Can you work these out from the model? Positions are in its coordinate system, mm. Face numbers are marked on the shaded views. Give positions to 0.01 mm unless a question says otherwise; leave off trailing zeros. Write each loop counter-clockwise with the first axis right and the second up, starting at its lowest first coordinate (ties: lowest second). Pieces come first, ordered by that corner, then holes.
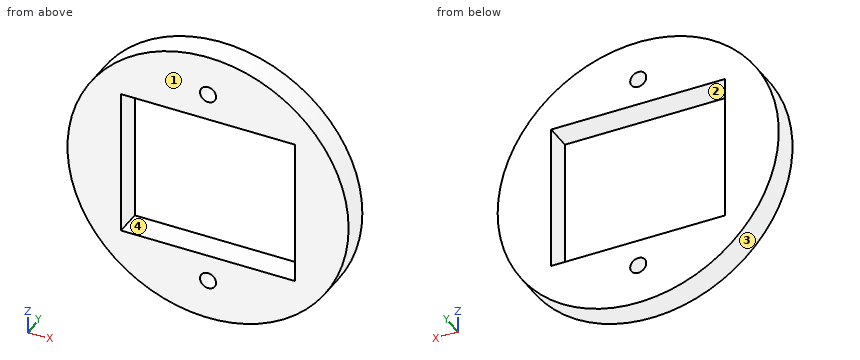
```python
from build123d import *

# Parameters (mm, degrees)
SKETCH1_R           = 26.67
SKETCH1_R_2         = 1.524
BOSS_EXTRUDE2_DEPTH = 5.08
SKETCH4_W           = 33.02
SKETCH4_H           = 27.94
CUT_EXTRUDE1_DEPTH  = 6.08


with BuildPart() as part:
    # Sketch1 → Boss-Extrude2 (new body)
    with BuildSketch(Plane(origin=(0, 0, 0), x_dir=(1, 0, 0), z_dir=(0, 1, 0))):
        Circle(SKETCH1_R)
        with Locations((0, -19.05)):
            Circle(SKETCH1_R_2, mode=Mode.SUBTRACT)
        with Locations((0, 19.05)):
            Circle(SKETCH1_R_2, mode=Mode.SUBTRACT)
    extrude(amount=BOSS_EXTRUDE2_DEPTH)

    # Sketch4 → Cut-Extrude1 (cut, through all)
    with BuildSketch(Plane(origin=(0, 5.08, 0), x_dir=(1, 0, 0), z_dir=(0, 1, 0))):
        Rectangle(SKETCH4_W, SKETCH4_H)
    extrude(amount=-CUT_EXTRUDE1_DEPTH, mode=Mode.SUBTRACT)


solid = part.part
```
1) Suppose I cut it at D-D on z = -7.5. Write out the boundary of the cut face in (x, y), plus the area to 3 significant figures.
Values follow:
outline: (-25.59, 0) - (-16.51, 0) - (-16.51, 5.08) - (-25.59, 5.08) - close; (16.51, 0) - (25.59, 0) - (25.59, 5.08) - (16.51, 5.08) - close
area: 92.3 mm2
2) For pin 1 Ø2.5 at (x, y) = (2, 2.5) entering from -Z; pin 2 Ø2.5 at (y, z) = (3.5, -5.5) entering from +X, each with a flat end and sliding along its axis, tell me the tip position at first contact or that it passes through.
Values follow:
pin 1: stops at z = -26.66
pin 2: stops at x = 26.33
3) Suppose I cut it at B-B on y = 3.3. Write out the boundary of the cut face in (x, z).
Values follow:
outline: circle Ø53.34 at (0, 0); hole (-16.51, -13.97) - (16.51, -13.97) - (16.51, 13.97) - (-16.51, 13.97) - close; hole circle Ø3.05 at (0, -19.05); hole circle Ø3.05 at (0, 19.05)
4) If we mould it in two halves opening along Z, with no side actions, what happens to the marked faces 1, 2, 3 and 4? For each: +Z half, -Z half, draft (parallel to the pull), parting line (faces both ways), or undercut.
Values follow:
face 1: draft
face 2: undercut
face 3: parting line
face 4: undercut
5) Suppose I cut it at A-A on z = 0. Write out the boundary of the cut face in (x, y), plus the area to 3 significant figures.
Values follow:
outline: (-26.67, 0) - (-16.51, 0) - (-16.51, 5.08) - (-26.67, 5.08) - close; (16.51, 0) - (26.67, 0) - (26.67, 5.08) - (16.51, 5.08) - close
area: 103 mm2
6) Please list where these lines run through material, in increasing order: L1, parallel to Z at x = 0, y = 2.65; L2, parallel to Z at x = 7, y = 3.5; L3, parallel to X at y = 0.55, z = 5.
Values follow:
L1: z = -26.67 to -20.57, -17.53 to -13.97, 13.97 to 17.53, 20.57 to 26.67
L2: z = -25.73 to -13.97, 13.97 to 25.73
L3: x = -26.2 to -16.51, 16.51 to 26.2
7) Suppose I cut it at C-C on x = 0. Write out the boundary of the cut face in (y, z).
Values follow:
outline: (0, -26.67) - (5.08, -26.67) - (5.08, -20.57) - (0, -20.57) - close; (0, -17.53) - (5.08, -17.53) - (5.08, -13.97) - (0, -13.97) - close; (0, 13.97) - (5.08, 13.97) - (5.08, 17.53) - (0, 17.53) - close; (0, 20.57) - (5.08, 20.57) - (5.08, 26.67) - (0, 26.67) - close
